Geometry: see drawing. Coordinates: mm, zero at the bounding-box minimum. Coordinates: 2 decimals unless noted, no trailing zeros. Order: outer loops, then holes, each group sorted by start corner. A loop starts at its lowest first (then second) coordinate and runs counter-clockwise, first axis right, second up. Notation, with made-up numbers: (67.5, 1.5) -> (114.5, 1.5) arc R10 cw to (114.5, 12.5) -> close; hole circle Ø9 at (40.5, -12.75). An arc over 180 degrees is marked (long way). Write each question's results on one line, items separated by ' | '.
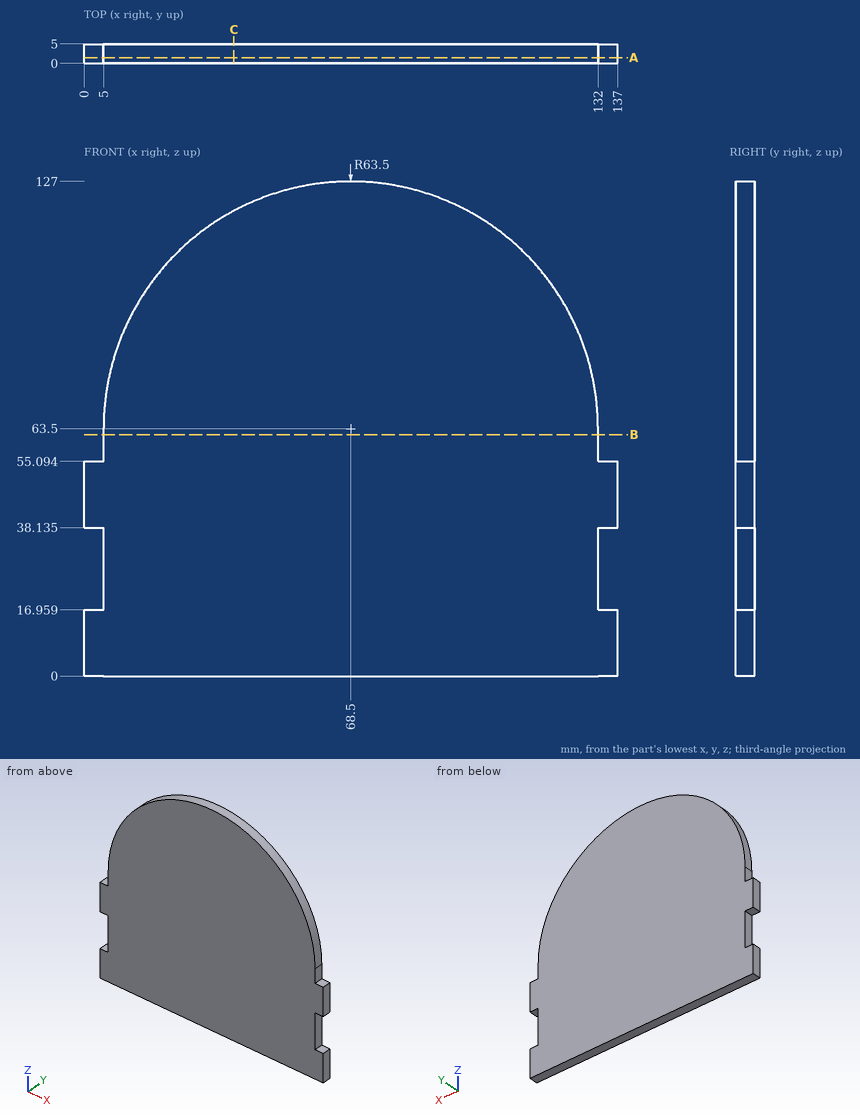
(1) Line query: line 1 along X through (y, z) = (1.45, 29.5); line 2 along Z through (x, y) = (68.5, 4.05); line 3 along Z through (x, y) = (57, 4.25). Output: solid intervals per line, ascending. Write a range as from..to.
Return value:
line 1: 5..132 | line 2: 0..127 | line 3: 0..125.95
(2) Cut plane B-B, the plane z = 62. Return loops of the section in (x, y), plus the area to 3 significant figures.
Return value:
outline: (5, 0) -> (132, 0) -> (132, 5) -> (5, 5) -> close | area: 635 mm2
(3) Cut plane A-A, the plane y = 1.5. Return loops of the section in (x, z) (1 decimal), plus the area to 3 significant figures.
Return value:
outline: (0, 0) -> (137, 0) -> (137, 17) -> (132, 17) -> (132, 38.1) -> (137, 38.1) -> (137, 55.1) -> (132, 55.1) -> (132, 63.5) arc R63.5 ccw to (5, 63.5) -> (5, 55.1) -> (0, 55.1) -> (0, 38.1) -> (5, 38.1) -> (5, 17) -> (0, 17) -> close | area: 14,700 mm2
(4) Cut plane C-C, the plane x = 38.5. Return loops of the section in (y, z).
Return value:
outline: (0, 0) -> (5, 0) -> (5, 119.47) -> (0, 119.47) -> close
(5) Pin query (flat end, axial travel): P1, Ø2.5, axis at x = 133.5, y = 3, coming from the +Z side; P2, Ø1.5, axis at y = 3, z = 31, coming from the -X side. Return the tip coordinate at first contact, or that it passes through.
Return value:
P1: z = 55.09 | P2: x = 5
